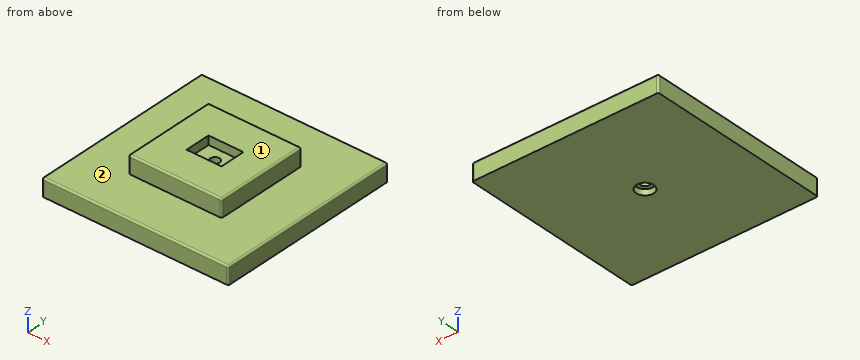
```python
from build123d import *

# Parameters (mm, degrees)
SKETCH1_W           = 160
SKETCH1_H           = 160
SKETCH1_W_2         = 80
SKETCH1_H_2         = 80
BOSS_EXTRUDE1_DEPTH = 15
SKETCH1_5_W         = 80
SKETCH1_5_H         = 80
BOSS_EXTRUDE2_DEPTH = 30
BOSS_EXTRUDE3_DEPTH = 22.5
SKETCH2_R           = 4
CUT_EXTRUDE2_DEPTH  = 22.5
SKETCH3_R           = 7.5
CUT_EXTRUDE3_DEPTH  = 5
FILLET1_R           = 1.5


with BuildPart() as part:
    # Sketch1 → Boss-Extrude1 (new body)
    with BuildSketch(Plane.XY):
        with Locations((80, 80)):
            Rectangle(SKETCH1_W, SKETCH1_H)
        with Locations((80, 80)):
            Rectangle(SKETCH1_W_2, SKETCH1_H_2, mode=Mode.SUBTRACT)
    extrude(amount=BOSS_EXTRUDE1_DEPTH)

    # Sketch1_5 → Boss-Extrude2 (add)
    with BuildSketch(Plane.XY):
        with Locations((80, 80)):
            Rectangle(SKETCH1_5_W, SKETCH1_5_H)
        Polygon((65, 91), (65, 69), (80, 69), (95, 69), (95, 91), align=None, mode=Mode.SUBTRACT)
    extrude(amount=BOSS_EXTRUDE2_DEPTH)

    # Sketch1_6 → Boss-Extrude3 (add)
    with BuildSketch(Plane.XY):
        Polygon((80, 91), (80, 80), (80, 69), (95, 69), (95, 91), align=None)
        Polygon((80, 69), (80, 80), (80, 91), (65, 91), (65, 69), align=None)
    extrude(amount=BOSS_EXTRUDE3_DEPTH)

    # Sketch2 → Cut-Extrude2 (cut)
    with BuildSketch(Plane.XY.offset(22.5)):
        with Locations((80, 80)):
            Circle(SKETCH2_R)
    extrude(amount=-CUT_EXTRUDE2_DEPTH, mode=Mode.SUBTRACT)

    # Sketch3 → Cut-Extrude3 (cut)
    with BuildSketch(Plane(origin=(0, 0, 0), x_dir=(-1, 0, 0), z_dir=(0, 0, -1))):
        with Locations((-80, 80)):
            Circle(SKETCH3_R)
    extrude(amount=-CUT_EXTRUDE3_DEPTH, mode=Mode.SUBTRACT)

    # Fillet1
    fillet1_edges = [part.edges().sort_by_distance(p)[0] for p in [
        (160, 80, 15),
        (80, 160, 15),
        (0, 0, 7.5),
        (0, 160, 7.5),
        (160, 160, 7.5),
        (160, 0, 7.5),
        (0, 80, 15),
        (120, 40, 22.5),
        (120, 80, 30),
        (120, 120, 22.5),
        (80, 120, 30),
        (40, 120, 22.5),
        (40, 40, 22.5),
        (40, 80, 30),
        (80, 40, 30),
        (80, 0, 15),
    ]]
    fillet(fillet1_edges, radius=FILLET1_R)


solid = part.part
```
Build history of the part. All positions in model axes, mm. Face numbers are marked on the shaded views. A direction names the side the tool comes from. Round coordinates to 2 decimals unless told otherwise and drop trailing zeros. Write each loop counter-clockwise with the first axis right and the second up, starting at its lowest first coordinate (ties: lowest second). Pieces come first, ordered by that corner, then holes. Notation, with made-up numbers: (-29.75, 75.25) -> (-15.75, 75.25) arc R16 cw to (-15.75, 83.25) -> close; hole circle Ø5 at (-13.75, 29.5). An arc over 180 degrees is marked (long way). Put each result on its own line as item: value.
Item 1: Slice it at D-D, the plane y = 98. Give the cut face in (x, z).
Here are the results:
outline: (0, 0) -> (160, 0) -> (160, 13.5) arc R1.5 ccw to (158.5, 15) -> (120, 15) -> (120, 28.5) arc R1.5 ccw to (118.5, 30) -> (41.5, 30) arc R1.5 ccw to (40, 28.5) -> (40, 15) -> (1.5, 15) arc R1.5 ccw to (0, 13.5) -> close
Item 2: Slice it at A-A, the plane x = 80. Give the cut face in (y, z).
Here are the results:
outline: (0, 0) -> (72.5, 0) -> (72.5, 5) -> (76, 5) -> (76, 22.5) -> (69, 22.5) -> (69, 30) -> (41.5, 30) arc R1.5 ccw to (40, 28.5) -> (40, 15) -> (1.5, 15) arc R1.5 ccw to (0, 13.5) -> close; (84, 5) -> (87.5, 5) -> (87.5, 0) -> (160, 0) -> (160, 13.5) arc R1.5 ccw to (158.5, 15) -> (120, 15) -> (120, 28.5) arc R1.5 ccw to (118.5, 30) -> (91, 30) -> (91, 22.5) -> (84, 22.5) -> close
Item 3: Tool access for the marked faces 1 and 2: list every direction of +Z, -Z, +X, -X, +Y, -Y with a clear straight run to the whole face (end or side of a thin tool).
Here are the results:
face 1: +Z, +X, -X, +Y, -Y
face 2: +Z
Item 4: Wall check: probe 1 along Y at (x, z) = (80, 2.1); probe 2 along Y at (x, z) = (80.5, 25); probe 3 along X at (y, z) = (90, 18.25). Give the ranges that are in metal, low to high. Write a range as from..to.
Here are the results:
probe 1: y = 0..72.5, 87.5..160
probe 2: y = 40..69, 91..120
probe 3: x = 40..120
Item 5: Slice it at B-B, the plane z = 25. Give the cut face in (x, y), plus the area to 3 significant figures.
Here are the results:
outline: (40, 41.5) arc R1.5 ccw to (41.5, 40) -> (118.5, 40) arc R1.5 ccw to (120, 41.5) -> (120, 118.5) arc R1.5 ccw to (118.5, 120) -> (41.5, 120) arc R1.5 ccw to (40, 118.5) -> close; hole (65, 69) -> (95, 69) -> (95, 91) -> (65, 91) -> close
area: 5,740 mm^2
Item 6: Flat gauge pins, fed straight in: P1, Ø4, axis at x = 18.5, y = 69.5, coming from the +Z side; P2, Ø11, axis at x = 91, z = 20, coming from the +Y side; P3, Ø2, axis at x = 83, z = 27, coming from the -Y side; P4, Ø6.5, axis at x = 80, y = 80, coming from the -Z side. Where does each tip first touch, or does it go through?
Here are the results:
P1: stops at z = 15
P2: stops at y = 159.62
P3: stops at y = 40
P4: passes through
Item 7: Slice it at C-C, the plane y = 80. Give the cut face in (x, z).
Here are the results:
outline: (0, 0) -> (72.5, 0) -> (72.5, 5) -> (76, 5) -> (76, 22.5) -> (65, 22.5) -> (65, 30) -> (41.5, 30) arc R1.5 ccw to (40, 28.5) -> (40, 15) -> (1.5, 15) arc R1.5 ccw to (0, 13.5) -> close; (84, 5) -> (87.5, 5) -> (87.5, 0) -> (160, 0) -> (160, 13.5) arc R1.5 ccw to (158.5, 15) -> (120, 15) -> (120, 28.5) arc R1.5 ccw to (118.5, 30) -> (95, 30) -> (95, 22.5) -> (84, 22.5) -> close
